Read the model definition and answer for the solid it produces. Units are mm, in the model's axes. Face numbers are marked on the shaded views. A direction names the side the tool comes from. Coordinates: 2 decimals unless noted, no trailing zeros. Write each loop counter-clockwise with the first axis right and the second up, starting at its lowest first coordinate (ties: lowest second). Pieces come first, ordered by that corner, then holes.
(1) Straight lines are drawn through the part: line 1 along X through (y, z) = (0.5, 3.75); line 2 along Y through (x, z) = (0, 1.2); line 3 along X through (y, z) = (11, 13.5). For each, find the intervals that lie inside material, in ascending order.
(2) Given pin 1 (8 mm diameter, centred on x = -27.5, z = 16.5, fed in from +Y); pin 2 (4 mm diameter, centred on x = 47, z = 17.5, fed in from +Y); pin 3 (3 mm diameter, centred on x = -24, z = 14.5, fed in from -Y), each flat-ended and moving along its own axis, determine where each tip first touches the part or whether it passes through.
(3) Which of the six approach directions +Z, -Z, +X, -X, +Y, -Y give full straight-line access (tool end or side, diameter ignored) to the marked faces 4, 5 and 6?
(4) Determine the mould class of the marked faces 1, 2 and 3 for opening direction X: pulls with the +X half, pulls with the -X half, needs draft (parallel to the pull), parting line crosses it, or undercut.
(5) The part is cut by section A-A, the plane y = 0. Determine the outline of the cut face in (x, z).
(6) The part is cut by section D-D, the plane y = -16.5. State how many separate pieces and enclosed holes the cut face has, and give its area (3 significant figures).
(7) The part is cut by section C-C, the plane x = 0. Determine the outline of the cut face in (y, z).
(8) The part is cut by section B-B, the plane z = 17.75. Determine the outline of the cut face in (x, y).
```python
from build123d import *

# Parameters (mm, degrees)
ESQUISSE1_R                  = 60
BOSS_EXTRU_1_DEPTH           = 25
ENL_V_MAT_EXTRU_1_DEPTH      = 89.459030065
ENL_V_MAT_EXTRU_1_DEPTH_BACK = 89.459030065
ESQUISSE2_W                  = 10
ESQUISSE2_H                  = 50
CHANFREIN1_SIZE              = 5
ENL_V_MAT_EXTRU_2_DEPTH      = 89.459030065
ENL_V_MAT_EXTRU_2_DEPTH_BACK = 89.459030065
ESQUISSE3_R                  = 5
ESQUISSE4_R                  = 18
ENL_V_MAT_EXTRU_3_DEPTH      = 4


with BuildPart() as part:
    # Esquisse1 → Boss.-Extru.1 (new body)
    with BuildSketch(Plane.XY):
        Circle(ESQUISSE1_R)
    extrude(amount=BOSS_EXTRU_1_DEPTH)

    # Esquisse2 → Enlèv. mat.-Extru.1 (cut, two sides: drawn at the far end of the back side and taken through both)
    with BuildSketch(Plane.XY.offset(25).offset(-ENL_V_MAT_EXTRU_1_DEPTH_BACK)):
        with Locations((-25, 0)):
            Rectangle(ESQUISSE2_W, ESQUISSE2_H)
        with Locations((25, 0)):
            Rectangle(ESQUISSE2_W, ESQUISSE2_H)
    extrude(amount=ENL_V_MAT_EXTRU_1_DEPTH + ENL_V_MAT_EXTRU_1_DEPTH_BACK, mode=Mode.SUBTRACT)

    # Chanfrein1
    chanfrein1_edges = [part.edges().sort_by_distance(p)[0] for p in [
        (-60, 0, 25),
    ]]
    chamfer(chanfrein1_edges, length=CHANFREIN1_SIZE)

    # Esquisse3 → Enlèv. mat.-Extru.2 (cut, two sides: drawn at the far end of the back side and taken through both)
    with BuildSketch(Plane.XY.offset(25).offset(-ENL_V_MAT_EXTRU_2_DEPTH_BACK)):
        Circle(ESQUISSE3_R)
    extrude(amount=ENL_V_MAT_EXTRU_2_DEPTH + ENL_V_MAT_EXTRU_2_DEPTH_BACK, mode=Mode.SUBTRACT)

    # Esquisse4 → Enlèv. mat.-Extru.3 (cut)
    with BuildSketch(Plane(origin=(0, 0, 0), x_dir=(-1, 0, 0), z_dir=(0, 0, -1))):
        Circle(ESQUISSE4_R)
    extrude(amount=-ENL_V_MAT_EXTRU_3_DEPTH, mode=Mode.SUBTRACT)


solid = part.part
```
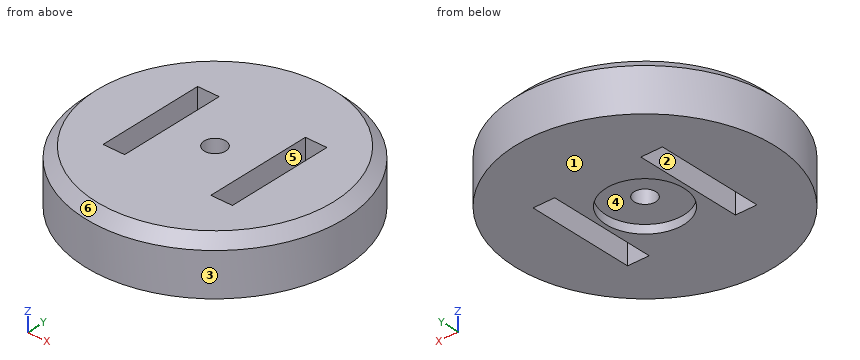
Computed:
1. line 1: x = -60 to -30, -20 to -17.99, 17.99 to 20, 30 to 60
1. line 2: y = -60 to -18, 18 to 60
1. line 3: x = -58.98 to -30, -20 to 20, 30 to 58.98
2. pin 1: stops at y = 55.21
2. pin 2: stops at y = 39.69
2. pin 3: stops at y = -55.62
3. face 4: -Z
3. face 5: +Z, -Z
3. face 6: +Z
4. face 1: needs draft
4. face 2: undercut
4. face 3: parting line crosses it
5. outline: (-60, 0) - (-30, 0) - (-30, 25) - (-55, 25) - (-60, 20) - close; (-20, 0) - (-18, 0) - (-18, 4) - (-5, 4) - (-5, 25) - (-20, 25) - close; (5, 4) - (18, 4) - (18, 0) - (20, 0) - (20, 25) - (5, 25) - close; (30, 0) - (60, 0) - (60, 20) - (55, 25) - (30, 25) - close
6. separate pieces: 3
6. enclosed holes: 0
6. area: 2,300 mm2
7. outline: (-60, 0) - (-18, 0) - (-18, 4) - (-5, 4) - (-5, 25) - (-55, 25) - (-60, 20) - close; (5, 4) - (18, 4) - (18, 0) - (60, 0) - (60, 20) - (55, 25) - (5, 25) - close
8. outline: circle Ø120 at (0, 0); hole (-30, -25) - (-20, -25) - (-20, 25) - (-30, 25) - close; hole circle Ø10 at (0, 0); hole (20, -25) - (30, -25) - (30, 25) - (20, 25) - close
